```python
from build123d import *

# Parameters (mm, degrees)
SKETCH1_R           = 1.5
BOSS_EXTRUDE1_DEPTH = 5
SKETCH3_R           = 10.5
CUT_EXTRUDE2_DEPTH  = 3.5
SKETCH4_W           = 25
SKETCH4_H           = 8.349364905
BOSS_EXTRUDE2_DEPTH = 40
FILLET1_R           = 4
SKETCH5_R           = 2.35
CUT_EXTRUDE3_DEPTH  = 6


with BuildPart() as part:
    # Sketch1 → Boss-Extrude1 (new body)
    # profile 1 of 5: a face of its own
    with BuildSketch(Plane.XY):
        with BuildLine():
            ThreePointArc((-12.5, 21.650635095), (-25, 0), (-12.5, -21.650635095))
            Line((-12.5, -21.650635095), (-12.5, 21.650635095))
        make_face()
    # profile 2 of 5: a face of its own
    with BuildSketch(Plane.XY):
        with BuildLine():
            Line((-12.5, 21.650635095), (-12.5, -21.650635095))
            ThreePointArc((-12.5, -21.650635095), (0, -25), (12.5, -21.650635095))
            Line((12.5, -21.650635095), (12.5, 21.650635095))
            ThreePointArc((12.5, 21.650635095), (0, 25), (-12.5, 21.650635095))
        make_face()
        with Locations((0, -7)):
            Circle(SKETCH1_R, mode=Mode.SUBTRACT)
        with Locations((7, 0)):
            Circle(SKETCH1_R, mode=Mode.SUBTRACT)
        with Locations((-7, 0)):
            Circle(SKETCH1_R, mode=Mode.SUBTRACT)
        Circle(SKETCH1_R, mode=Mode.SUBTRACT)
        with Locations((0, 7)):
            Circle(SKETCH1_R, mode=Mode.SUBTRACT)
    # profile 3 of 5: a face of its own
    with BuildSketch(Plane.XY):
        with BuildLine():
            Line((-12.5, 30), (-12.5, 21.650635095))
            ThreePointArc((-12.5, 21.650635095), (0, 25), (12.5, 21.650635095))
            Line((12.5, 21.650635095), (12.5, 30))
            Line((12.5, 30), (-12.5, 30))
        make_face()
    # profile 4 of 5: a face of its own
    with BuildSketch(Plane.XY):
        with BuildLine():
            Line((-12.5, -21.650635095), (-12.5, -30))
            Line((-12.5, -30), (12.5, -30))
            Line((12.5, -30), (12.5, -21.650635095))
            ThreePointArc((12.5, -21.650635095), (0, -25), (-12.5, -21.650635095))
        make_face()
    # profile 5 of 5: a face of its own
    with BuildSketch(Plane.XY):
        with BuildLine():
            Line((12.5, 21.650635095), (12.5, -21.650635095))
            ThreePointArc((12.5, -21.650635095), (21.650635095, -12.5), (25, 0))
            ThreePointArc((25, 0), (21.650635095, 12.5), (12.5, 21.650635095))
        make_face()
    extrude(amount=BOSS_EXTRUDE1_DEPTH)

    # Sketch3 → Cut-Extrude2 (cut)
    with BuildSketch(Plane(origin=(0, 0, 0), x_dir=(-1, 0, 0), z_dir=(0, 0, -1))):
        Circle(SKETCH3_R)
    extrude(amount=-CUT_EXTRUDE2_DEPTH, mode=Mode.SUBTRACT)

    # Sketch4 → Boss-Extrude2 (add)
    with BuildSketch(Plane.XY.offset(5)):
        with Locations((0, 25.825317548)):
            Rectangle(SKETCH4_W, SKETCH4_H)
        with Locations((0, -25.825317548)):
            Rectangle(SKETCH4_W, SKETCH4_H)
    extrude(amount=BOSS_EXTRUDE2_DEPTH)

    # Fillet1
    fillet1_edges = [part.edges().sort_by_distance(p)[0] for p in [
        (-12.5, 30, 22.5),
        (12.5, 30, 22.5),
        (12.5, -30, 22.5),
        (-12.5, -30, 22.5),
        (-12.5, 21.650635095, 25),
        (12.5, 21.650635095, 25),
        (-12.5, -21.650635095, 25),
        (12.5, -21.650635095, 25),
    ]]
    fillet(fillet1_edges, radius=FILLET1_R)

    # Sketch5 → Cut-Extrude3 (cut)
    with BuildSketch(Plane.XY.offset(45)):
        with Locations((-7.5, 25.825317547)):
            Circle(SKETCH5_R)
        with Locations(Location((7.5, 25.825317547, 0), (0, 0, 180))):
            Circle(SKETCH5_R)
        with Locations((7.5, -25.825317547)):
            Circle(SKETCH5_R)
        with Locations(Location((-7.5, -25.825317547, 0), (0, 0, 180))):
            Circle(SKETCH5_R)
    extrude(amount=-CUT_EXTRUDE3_DEPTH, mode=Mode.SUBTRACT)


solid = part.part
```
CAD build for the part. Positions are in the model's coordinates, mm. A direction names the side the tool comes from. Give positions to 0.01 mm unless a question says otherwise; leave off trailing zeros. Write each loop counter-clockwise with the first axis right and the second up, starting at its lowest first coordinate (ties: lowest second). Pieces come first, ordered by that corner, then holes. Notation, with made-up numbers: M 86.25,80.5 L 129.25,80.5 A21 cw 129.25,85.5 Z; hole C -28,88.25 d1. An arc over 180 degrees is marked long. Return JSON: item names as keys, results as strings. Group by question number.
(1) Flat gauge pins, fed straight in: pin 1 Ø3.5 at (x, y) = (0, 0) entering from -Z; pin 2 Ø5 at (y, z) = (-24.5, 19) entering from -X; pin 3 Ø4 at (x, y) = (-7.5, 25.83) entering from +Z; pin 4 Ø1.8 at (x, y) = (0, 7) entering from -Z. Where does each tip first touch, or does it go through?
(2) Band-saw the part on C-C (y = 7). Give the cut face in (x, z).
(3) Band-saw the part on B-B (z = 9). Give the cut face in (x, y), and give its area (3 significant figures).
(4) 3-axis set-ups, long thin cutter, end or side, ignore diameter. For faces 4 (the face through (-10, 3.2, 1.7)), 5 (the face through (-11.297, -22.791, 25.28)), 6 (the face through (7, -26, 39)): which of +Z, -Z, +X, -X, +Y, -Y reach the whole face in a straight line?
(5) Mould opens along Y. For faces 1 (the face through (-25, 0, 2)), 2 (the face through (0, -30, 22)), 3 (the face through (0, -21.651, 25)) say: pulls with the +Y half, pulls with the -Y half, needs draft (parallel to the pull), parting line crosses it, or undercut.
(6) Drill centre lines: L1, parallel to Y at x = -7, z = 4.4; L2, parallel to Y at x = 2, z = 9; L3, parallel to Y at x = -7, z = 42. Where is each one in solid material? Low to high. Write a range as [from, to].
(7) Band-saw the part on D-D (z = 41). Give the cut face in (x, y).
(8) Band-saw the part on A-A (x = 0). Give the cut face in (y, z), and give its area (3 significant figures).
Entries:
{
 "1": {"pin 1": "stops at z = 3.5", "pin 2": "stops at x = -12.5", "pin 3": "stops at z = 39", "pin 4": "passes through"},
 "2": {"outline": "M -24,0 L -7.83,0 L -7.83,3.5 L -1.5,3.5 L -1.5,5 L -24,5 Z; M 1.5,3.5 L 7.83,3.5 L 7.83,0 L 24,0 L 24,5 L 1.5,5 Z"},
 "3": {"outline": "M -12.5,-26 A4 ccw -8.5,-30 L 8.5,-30 A4 ccw 12.5,-26 L 12.5,-25.65 A4 ccw 8.5,-21.65 L -8.5,-21.65 A4 ccw -12.5,-25.65 Z; M -12.5,25.65 A4 ccw -8.5,21.65 L 8.5,21.65 A4 ccw 12.5,25.65 L 12.5,26 A4 ccw 8.5,30 L -8.5,30 A4 ccw -12.5,26 Z", "area": "390 mm^2"},
 "4": {"face 4": "-Z", "face 5": "+Z, -X", "face 6": "+Z"},
 "5": {"face 1": "parting line crosses it", "face 2": "pulls with the -Y half", "face 3": "undercut"},
 "6": {"L1": "y = [-30, -1.5], [1.5, 30]", "L2": "y = [-30, -21.65], [21.65, 30]", "L3": "y = [-30, -28.12], [-23.53, -21.65], [21.65, 23.53], [28.12, 30]"},
 "7": {"outline": "M -12.5,-26 A4 ccw -8.5,-30 L 8.5,-30 A4 ccw 12.5,-26 L 12.5,-25.65 A4 ccw 8.5,-21.65 L -8.5,-21.65 A4 ccw -12.5,-25.65 Z; M -12.5,25.65 A4 ccw -8.5,21.65 L 8.5,21.65 A4 ccw 12.5,25.65 L 12.5,26 A4 ccw 8.5,30 L -8.5,30 A4 ccw -12.5,26 Z; hole C -7.5,-25.83 d4.7; hole C -7.5,25.83 d4.7; hole C 7.5,-25.83 d4.7; hole C 7.5,25.83 d4.7"},
 "8": {"outline": "M -30,0 L -10.5,0 L -10.5,3.5 L -8.5,3.5 L -8.5,5 L -21.65,5 L -21.65,45 L -30,45 Z; M -5.5,3.5 L -1.5,3.5 L -1.5,5 L -5.5,5 Z; M 1.5,3.5 L 5.5,3.5 L 5.5,5 L 1.5,5 Z; M 8.5,3.5 L 10.5,3.5 L 10.5,0 L 30,0 L 30,45 L 21.65,45 L 21.65,5 L 8.5,5 Z", "area": "881 mm^2"}
}
